```python
from build123d import *

# Parameters (mm, degrees)
SKETCH_1_W          = 132.5
SKETCH_1_H          = 73.1
EXTRUDE_1_DEPTH     = 48.2
SKETCH_3_W          = 122.5
SKETCH_3_H          = 43.2
CUT_EXTRUDE_1_DEPTH = 68.1
SKETCH_6_W          = 20
SKETCH_6_H          = 10
CUT_EXTRUDE_2_DEPTH = 5


with BuildPart() as part:
    # 草圖1 → 填料-伸長1 (new body)
    with BuildSketch(Plane(origin=(0, 0, 0), x_dir=(1, 0, 0), z_dir=(0, 1, 0))):
        Rectangle(SKETCH_1_W, SKETCH_1_H)
    extrude(amount=EXTRUDE_1_DEPTH)

    # 草圖3 → 除料-伸長1 (cut)
    with BuildSketch(Plane.XY.offset(36.55)):
        with Locations((0, 21.6)):
            Rectangle(SKETCH_3_W, SKETCH_3_H)
    extrude(amount=-CUT_EXTRUDE_1_DEPTH, mode=Mode.SUBTRACT)

    # 草圖6 → 除料-伸長2 (cut)
    with BuildSketch(Plane.ZY.offset(66.25)):
        with Locations((0, 38.2)):
            Rectangle(SKETCH_6_W, SKETCH_6_H)
    extrude(amount=-CUT_EXTRUDE_2_DEPTH, mode=Mode.SUBTRACT)


solid = part.part
```
Geometry check sheet. Reference: the model listing, model coordinates, mm. A direction names the side the tool comes from. Coordinates: 2 decimals unless noted, no trailing zeros. Order: outer loops, then holes, each group sorted by start corner. A loop starts at its lowest first (then second) coordinate and runs counter-clockwise, first axis right, second up.
Q1. Sectioned sample at A-A on z = -5. Record the cut outline in (x, y).
Reply:
outline: (-66.25, 0) - (-61.25, 0) - (-61.25, 33.2) - (-66.25, 33.2) - close; (-66.25, 43.2) - (61.25, 43.2) - (61.25, 0) - (66.25, 0) - (66.25, 48.2) - (-66.25, 48.2) - close
Q2. Sectioned sample at B-B on y = 39. Record the cut outline in (x, z).
Reply:
outline: (-66.25, -36.55) - (66.25, -36.55) - (66.25, 36.55) - (61.25, 36.55) - (61.25, -31.55) - (-61.25, -31.55) - (-61.25, -10) - (-66.25, -10) - close; (-66.25, 10) - (-61.25, 10) - (-61.25, 36.55) - (-66.25, 36.55) - close
Q3. Sectioned sample at D-D on x = 22. Record the cut outline in (y, z).
Reply:
outline: (0, -36.55) - (48.2, -36.55) - (48.2, 36.55) - (43.2, 36.55) - (43.2, -31.55) - (0, -31.55) - close
Q4. Sectioned sample at C-C on z = 29. Record the cut outline in (x, y), and give its area (3 significant figures).
Reply:
outline: (-66.25, 0) - (-61.25, 0) - (-61.25, 43.2) - (61.25, 43.2) - (61.25, 0) - (66.25, 0) - (66.25, 48.2) - (-66.25, 48.2) - close
area: 1,090 mm2
Q5. Tool access check on faces 1 (the face through (0, 45, 36.55)), 2 (the face through (61.25, 21, 3)), 3 (the face through (-64, 38, -10)). Record the directions out of +Z, -Z, +X, -X, +Y, -Y that give a thin tool (end or side, any length) a straight path to the whole face; none if there is none.
Reply:
face 1: +Z, +X, -X, +Y, -Y
face 2: +Z, -Y
face 3: -X
Q6. Thickness scan on probe 1 along X at (y, z) = (38.5, -26); probe 2 along Y at (x, z) = (29, -28); probe 3 along Z at (x, y) = (42.5, 27). Record the ranges inside material, lowest first.
Reply:
probe 1: x = -66.25 to -61.25, 61.25 to 66.25
probe 2: y = 43.2 to 48.2
probe 3: z = -36.55 to -31.55
Q7. Depth check by flat-ended pin: pin 1 Ø6 at (x, y) = (-11.5, 17) entering from +Z; pin 2 Ø2 at (x, z) = (7.5, 3.5) entering from -Y. Enter the tip coordinate at first touch or a pass-through.
Reply:
pin 1: stops at z = -31.55
pin 2: stops at y = 43.2
Q8. Draft check along X on faces 4 (the face through (-1, 22, -31.55)), 5 (the face through (-3, 43.2, 2)), 6 (the face through (66.25, 24, 1)), 7 (the face through (-64, 33.2, 0)). Enter one of: released by +X, released by -X, zero draft, split by the parting line, or undercut.
Reply:
face 4: undercut
face 5: undercut
face 6: released by +X
face 7: zero draft
